Part print with two shaded views. Sizes in mm from the minimum x, y, z corner. Round coordinates to 2 decimals unless told otherwise and drop trailing zeros. Write each loop counter-clockwise with the first axis right and the second up, starting at its lowest first coordinate (ties: lowest second). Pieces come first, ordered by that corner, then holes. Notation, with made-up numbers: (-17, 58.25) -> (-2, 58.25) arc R22 cw to (-2, 66.25) -> close; hole circle Ø10 at (60, 34.25). An arc over 180 degrees is marked (long way). Put each result on its own line as item: value. Start each with the question number.
1. Saw through at B-B on x = 5. List the corners of the cut face in (y, z).
2. Saw through at D-D on x = 25. List the corners of the cut face in (y, z), and give its area (3 significant figures).
3. Saw through at A-A on z = 20. List the corners of the cut face in (x, y), and give its area (3 significant figures).
4. Saw through at C-C on z = 35. List the corners of the cut face in (x, y), and give its area (3 significant figures).
5. Drill centre line: line 1 (Y direction, x = 42.5, z = 10.5). Where is it in solid material? Low to high. Write a range as from..to.
6. Flat gauge pin, fed straight in: P1, Ø1.5, axis at x = 18, z = 26.5, coming from the -Y side. Where does the tip first touch, or does it go through?
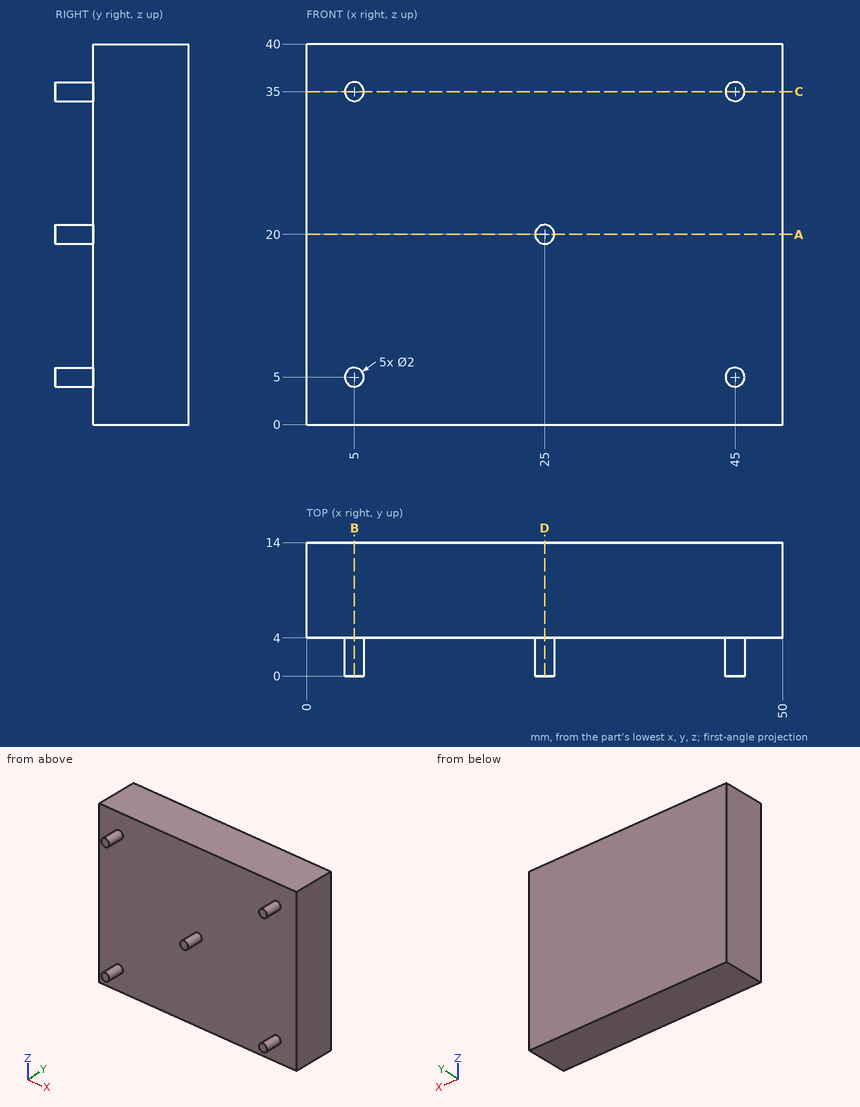
Return value:
1. outline: (0, 4) -> (4, 4) -> (4, 0) -> (14, 0) -> (14, 40) -> (4, 40) -> (4, 36) -> (0, 36) -> (0, 34) -> (4, 34) -> (4, 6) -> (0, 6) -> close
2. outline: (0, 19) -> (4, 19) -> (4, 0) -> (14, 0) -> (14, 40) -> (4, 40) -> (4, 21) -> (0, 21) -> close
2. area: 408 mm^2
3. outline: (0, 4) -> (24, 4) -> (24, 0) -> (26, 0) -> (26, 4) -> (50, 4) -> (50, 14) -> (0, 14) -> close
3. area: 508 mm^2
4. outline: (0, 4) -> (4, 4) -> (4, 0) -> (6, 0) -> (6, 4) -> (44, 4) -> (44, 0) -> (46, 0) -> (46, 4) -> (50, 4) -> (50, 14) -> (0, 14) -> close
4. area: 516 mm^2
5. line 1: y = 4..14
6. P1: stops at y = 4
